```python
from build123d import *

# Parameters (mm, degrees)
SKETCH_1_R      = 1.55
SKETCH_1_W      = 10
SKETCH_1_H      = 6.1
EXTRUDE_1_DEPTH = 6


with BuildPart() as part:
    # Эскиз1 → Бобышка-Вытянуть1 (new body)
    with BuildSketch(Plane(origin=(0, 0, 0), x_dir=(1, 0, 0), z_dir=(0, 1, 0))):
        with BuildLine():
            Line((40.261608154, 29.273839185), (40.011608154, 23.273839185))
            Line((40.011608154, 23.273839185), (14.511608154, 23.273839185))
            Line((14.511608154, 23.273839185), (14.261608154, 29.273839185))
            Line((14.261608154, 29.273839185), (4.261608154, 29.273839185))
            Line((4.261608154, 29.273839185), (4.011608154, 23.273839185))
            Line((4.011608154, 23.273839185), (-1.188391846, 23.273839185))
            Line((-1.188391846, 23.273839185), (-1.188391846, 16.473839185))
            Line((-1.188391846, 16.473839185), (0.011608154, 16.473839185))
            Line((0.011608154, 16.473839185), (0.011608154, 14.273839185))
            Line((0.011608154, 14.273839185), (-1.188391846, 14.273839185))
            Line((-1.188391846, 14.273839185), (-1.188391846, 12.773839185))
            Line((-1.188391846, 12.773839185), (-4.288391846, 12.773839185))
            Line((-4.288391846, 12.773839185), (-4.288391846, 14.273839185))
            Line((-4.288391846, 14.273839185), (-5.488391846, 14.273839185))
            Line((-5.488391846, 14.273839185), (-5.488391846, 16.473839185))
            Line((-5.488391846, 16.473839185), (-4.288391846, 16.473839185))
            Line((-4.288391846, 16.473839185), (-4.288391846, 23.273839185))
            Line((-4.288391846, 23.273839185), (-9.488391846, 23.273839185))
            Line((-9.488391846, 23.273839185), (-9.738391846, 29.273839185))
            Line((-9.738391846, 29.273839185), (-19.738391846, 29.273839185))
            Line((-19.738391846, 29.273839185), (-19.988391846, 23.273839185))
            Line((-19.988391846, 23.273839185), (-24.238391846, 23.273839185))
            Line((-24.238391846, 23.273839185), (-24.238391846, 17.273839185))
            ThreePointArc((-24.238391846, 17.273839185), (-25.409964721, 14.44541206), (-28.238391846, 13.273839185))
            Line((-28.238391846, 13.273839185), (-59.238391846, 13.273839185))
            Line((-59.238391846, 13.273839185), (-59.238391846, 11.323839185))
            Line((-59.238391846, 11.323839185), (-71.238391846, 11.273839185))
            Line((-71.238391846, 11.273839185), (-71.238391846, 1.273839185))
            Line((-71.238391846, 1.273839185), (-59.238391846, 1.223839185))
            Line((-59.238391846, 1.223839185), (-59.238391846, -1.176160815))
            Line((-59.238391846, -1.176160815), (-52.438391846, -1.176160815))
            Line((-52.438391846, -1.176160815), (-52.438391846, 0.023839185))
            Line((-52.438391846, 0.023839185), (-50.238391846, 0.023839185))
            Line((-50.238391846, 0.023839185), (-50.238391846, -1.176160815))
            Line((-50.238391846, -1.176160815), (-48.738391846, -1.176160815))
            Line((-48.738391846, -1.176160815), (-48.738391846, -4.276160815))
            Line((-48.738391846, -4.276160815), (-50.238391846, -4.276160815))
            Line((-50.238391846, -4.276160815), (-50.238391846, -5.476160815))
            Line((-50.238391846, -5.476160815), (-52.438391846, -5.476160815))
            Line((-52.438391846, -5.476160815), (-52.438391846, -4.276160815))
            Line((-52.438391846, -4.276160815), (-59.238391846, -4.276160815))
            Line((-59.238391846, -4.276160815), (-59.238391846, -6.676160815))
            Line((-59.238391846, -6.676160815), (-71.238391846, -6.726160815))
            Line((-71.238391846, -6.726160815), (-71.238391846, -16.726160815))
            Line((-71.238391846, -16.726160815), (-59.238391846, -16.776160815))
            Line((-59.238391846, -16.776160815), (-59.238391846, -18.726160815))
            Line((-59.238391846, -18.726160815), (-28.238391846, -18.726160815))
            ThreePointArc((-28.238391846, -18.726160815), (-25.409964721, -19.897733691), (-24.238391846, -22.726160815))
            Line((-24.238391846, -22.726160815), (-24.238391846, -28.726160815))
            Line((-24.238391846, -28.726160815), (-19.988391846, -28.726160815))
            Line((-19.988391846, -28.726160815), (-19.738391846, -34.726160815))
            Line((-19.738391846, -34.726160815), (-9.738391846, -34.726160815))
            Line((-9.738391846, -34.726160815), (-9.488391846, -28.726160815))
            Line((-9.488391846, -28.726160815), (-4.288391846, -28.726160815))
            Line((-4.288391846, -28.726160815), (-4.288391846, -21.926160815))
            Line((-4.288391846, -21.926160815), (-5.488391846, -21.926160815))
            Line((-5.488391846, -21.926160815), (-5.488391846, -19.726160815))
            Line((-5.488391846, -19.726160815), (-4.288391846, -19.726160815))
            Line((-4.288391846, -19.726160815), (-4.288391846, -18.226160815))
            Line((-4.288391846, -18.226160815), (-1.188391846, -18.226160815))
            Line((-1.188391846, -18.226160815), (-1.188391846, -19.726160815))
            Line((-1.188391846, -19.726160815), (0.011608154, -19.726160815))
            Line((0.011608154, -19.726160815), (0.011608154, -21.926160815))
            Line((0.011608154, -21.926160815), (-1.188391846, -21.926160815))
            Line((-1.188391846, -21.926160815), (-1.188391846, -28.726160815))
            Line((-1.188391846, -28.726160815), (4.011608154, -28.726160815))
            Line((4.011608154, -28.726160815), (4.261608154, -34.726160815))
            Line((4.261608154, -34.726160815), (14.261608154, -34.726160815))
            Line((14.261608154, -34.726160815), (14.511608154, -28.726160815))
            Line((14.511608154, -28.726160815), (40.011608154, -28.726160815))
            Line((40.011608154, -28.726160815), (40.261608154, -34.726160815))
            Line((40.261608154, -34.726160815), (50.261608154, -34.726160815))
            Line((50.261608154, -34.726160815), (50.511608154, -28.726160815))
            Line((50.511608154, -28.726160815), (55.711608154, -28.726160815))
            Line((55.711608154, -28.726160815), (55.711608154, -21.926160815))
            Line((55.711608154, -21.926160815), (54.511608154, -21.926160815))
            Line((54.511608154, -21.926160815), (54.511608154, -19.726160815))
            Line((54.511608154, -19.726160815), (55.711608154, -19.726160815))
            Line((55.711608154, -19.726160815), (55.711608154, -18.226160815))
            Line((55.711608154, -18.226160815), (58.811608154, -18.226160815))
            Line((58.811608154, -18.226160815), (58.811608154, -19.726160815))
            Line((58.811608154, -19.726160815), (60.011608154, -19.726160815))
            Line((60.011608154, -19.726160815), (60.011608154, -21.926160815))
            Line((60.011608154, -21.926160815), (58.811608154, -21.926160815))
            Line((58.811608154, -21.926160815), (58.811608154, -28.726160815))
            Line((58.811608154, -28.726160815), (64.011608154, -28.726160815))
            Line((64.011608154, -28.726160815), (64.261608154, -34.726160815))
            Line((64.261608154, -34.726160815), (74.261608154, -34.726160815))
            Line((74.261608154, -34.726160815), (74.511608154, -28.726160815))
            Line((74.511608154, -28.726160815), (78.761608154, -28.726160815))
            Line((78.761608154, -28.726160815), (78.761608154, -22.726160815))
            ThreePointArc((78.761608154, -22.726160815), (79.933181029, -19.897733691), (82.761608154, -18.726160815))
            Line((82.761608154, -18.726160815), (113.761608154, -18.726160815))
            Line((113.761608154, -18.726160815), (113.761608154, -16.776160815))
            Line((113.761608154, -16.776160815), (125.761608154, -16.726160815))
            Line((125.761608154, -16.726160815), (125.761608154, -6.726160815))
            Line((125.761608154, -6.726160815), (113.761608154, -6.676160815))
            Line((113.761608154, -6.676160815), (113.761608154, -4.276160815))
            Line((113.761608154, -4.276160815), (106.961608154, -4.276160815))
            Line((106.961608154, -4.276160815), (106.961608154, -5.476160815))
            Line((106.961608154, -5.476160815), (104.761608154, -5.476160815))
            Line((104.761608154, -5.476160815), (104.761608154, -4.276160815))
            Line((104.761608154, -4.276160815), (103.261608154, -4.276160815))
            Line((103.261608154, -4.276160815), (103.261608154, -1.176160815))
            Line((103.261608154, -1.176160815), (104.761608154, -1.176160815))
            Line((104.761608154, -1.176160815), (104.761608154, 0.023839185))
            Line((104.761608154, 0.023839185), (106.961608154, 0.023839185))
            Line((106.961608154, 0.023839185), (106.961608154, -1.176160815))
            Line((106.961608154, -1.176160815), (113.761608154, -1.176160815))
            Line((113.761608154, -1.176160815), (113.761608154, 1.223839185))
            Line((113.761608154, 1.223839185), (125.761608154, 1.273839185))
            Line((125.761608154, 1.273839185), (125.761608154, 11.273839185))
            Line((125.761608154, 11.273839185), (113.761608154, 11.323839185))
            Line((113.761608154, 11.323839185), (113.761608154, 13.273839185))
            Line((113.761608154, 13.273839185), (82.761608154, 13.273839185))
            ThreePointArc((82.761608154, 13.273839185), (79.933181029, 14.44541206), (78.761608154, 17.273839185))
            Line((78.761608154, 17.273839185), (78.761608154, 23.273839185))
            Line((78.761608154, 23.273839185), (74.511608154, 23.273839185))
            Line((74.511608154, 23.273839185), (74.261608154, 29.273839185))
            Line((74.261608154, 29.273839185), (64.261608154, 29.273839185))
            Line((64.261608154, 29.273839185), (64.011608154, 23.273839185))
            Line((64.011608154, 23.273839185), (58.811608154, 23.273839185))
            Line((58.811608154, 23.273839185), (58.811608154, 16.473839185))
            Line((58.811608154, 16.473839185), (60.011608154, 16.473839185))
            Line((60.011608154, 16.473839185), (60.011608154, 14.273839185))
            Line((60.011608154, 14.273839185), (58.811608154, 14.273839185))
            Line((58.811608154, 14.273839185), (58.811608154, 12.773839185))
            Line((58.811608154, 12.773839185), (55.711608154, 12.773839185))
            Line((55.711608154, 12.773839185), (55.711608154, 14.273839185))
            Line((55.711608154, 14.273839185), (54.511608154, 14.273839185))
            Line((54.511608154, 14.273839185), (54.511608154, 16.473839185))
            Line((54.511608154, 16.473839185), (55.711608154, 16.473839185))
            Line((55.711608154, 16.473839185), (55.711608154, 23.273839185))
            Line((55.711608154, 23.273839185), (50.511608154, 23.273839185))
            Line((50.511608154, 23.273839185), (50.261608154, 29.273839185))
            Line((50.261608154, 29.273839185), (40.261608154, 29.273839185))
        make_face()
        with Locations((-2.738391846, -2.726160815)):
            Circle(SKETCH_1_R, mode=Mode.SUBTRACT)
        with Locations((57.261608154, -2.726160815)):
            Circle(SKETCH_1_R, mode=Mode.SUBTRACT)
        with Locations((9.261608154, -2.726160815)):
            Rectangle(SKETCH_1_W, SKETCH_1_H, mode=Mode.SUBTRACT)
        with Locations((-14.738391846, -2.726160815)):
            Rectangle(SKETCH_1_W, SKETCH_1_H, mode=Mode.SUBTRACT)
        with Locations((45.261608154, -2.726160815)):
            Rectangle(SKETCH_1_W, SKETCH_1_H, mode=Mode.SUBTRACT)
        with Locations((69.261608154, -2.726160815)):
            Rectangle(SKETCH_1_W, SKETCH_1_H, mode=Mode.SUBTRACT)
    extrude(amount=EXTRUDE_1_DEPTH)


solid = part.part
```
Here's how the part is built. I have some questions about the finished solid (model axes, mm). A direction names the side the tool comes from. Coordinates: 2 decimals unless noted, no trailing zeros. Order: outer loops, then holes, each group sorted by start corner. A loop starts at its lowest first (then second) coordinate and runs counter-clockwise, first axis right, second up.
Item 1: Thinking about a two-plate mould opening in Z: for faces 1 (the face through (125.762, 3, -6)), 2 (the face through (-15, 3, 5.776)), 3 (the face through (-25.379, 2.958, -14.477)), which applies, pulls with the +Z half, pulls with the -Z half, needs draft (parallel to the pull), parting line crosses it, or undercut?
Response values:
face 1: needs draft
face 2: undercut
face 3: pulls with the -Z half
Item 2: If we section it at A-A, the plane x = -22: List the corners of the cut face in (y, z) for me.
Response values:
outline: (0, -23.27) - (6, -23.27) - (6, 28.73) - (0, 28.73) - close
Item 3: I'm going to push flat-ended pins straight in: pin 1 Ø1.1 at (x, y) = (105.5, 1.5) entering from -Z; pin 2 Ø3.5 at (x, z) = (57.26, 2.73) entering from +Y; pin 3 Ø2.5 at (y, z) = (3.5, 21.5) entering from -X; pin 4 Ø0.6 at (x, y) = (-5, 1.5) entering from +Z. Where does each tip first touch, or does it pass through?
Response values:
pin 1: stops at z = -13.27
pin 2: stops at y = 6
pin 3: stops at x = -25.1
pin 4: stops at z = 28.73
Item 4: I need wall thicknesses on probe 1 along X at (y, z) = (1.8, -17); probe 2 along X at (y, z) = (2.6, -13); probe 3 along Z at (x, y) = (110, 2.7). Which ranges of each line are inside material? Lowest first, please.
Response values:
probe 1: x = -24.25 to -4.29, -1.19 to 55.71, 58.81 to 78.77
probe 2: x = -59.24 to -4.29, -1.19 to 55.71, 58.81 to 113.76
probe 3: z = -13.27 to 1.18, 4.28 to 18.73
Item 5: If we section it at B-B, the plane y = 3.9: Give the number of separate pieces and of enclosed holes in the cut face, then the cut area to 3 significant figures.
Response values:
separate pieces: 1
enclosed holes: 6
area: 8,100 mm2
Item 6: Which directions (+Z, -Z, +X, -X, +Y, -Y) give clear straight access to the entire face, cutting with the end or side of a thin tool? Please do faces 4 (the face through (58.812, 3, 25)), 5 (the face through (69, 3, -29.274)), 6 (the face through (1, 3, -23.274)), 7 (the face through (98, 3, 18.726)), 8 (the face through (78.762, 3, -20)).
Response values:
face 4: +Z, +Y, -Y
face 5: -Z, +X, -X, +Y, -Y
face 6: -Z, +Y, -Y
face 7: +Z, +X, +Y, -Y
face 8: -Z, +X, +Y, -Y
